from build123d import *

# Parameters (mm, degrees)
SKETCH1_W           = 12.7
SKETCH1_H           = 12.7
BOSS_EXTRUDE1_DEPTH = 2.54
FILLET1_R           = 0.635
SHELL1_START        = 0.635
SHELL1_OUTLINE_W    = 1.905
SHELL1_OUTLINE_H    = 11.43
SHELL1_DEPTH        = 11.43
SKETCH2_R           = 2.54
BOSS_EXTRUDE2_DEPTH = 1.905
BOSS_EXTRUDE3_DEPTH = 0.00254


# Read off the part's stored shape, not the designer's step: Shell1
with BuildPart() as part:
    # Sketch1 → Boss-Extrude1 (new body)
    with BuildSketch(Plane(origin=(0, 0, 0), x_dir=(1, 0, 0), z_dir=(0, 1, 0))):
        with Locations((6.35, 6.35)):
            Rectangle(SKETCH1_W, SKETCH1_H)
    extrude(amount=BOSS_EXTRUDE1_DEPTH)

    # Fillet1
    fillet1_edges = [part.edges().sort_by_distance(p)[0] for p in [
        (0, 1.27, -12.7),
        (12.7, 1.27, -12.7),
        (12.7, 1.27, 0),
        (0, 1.27, 0),
    ]]
    fillet(fillet1_edges, radius=FILLET1_R)

    # Shell1 outline → Shell1 (cut)
    with BuildSketch(Plane.YZ.offset(SHELL1_START)):
        with Locations((0.9525, -6.35)):
            Rectangle(SHELL1_OUTLINE_W, SHELL1_OUTLINE_H)
    extrude(amount=SHELL1_DEPTH, mode=Mode.SUBTRACT)

    # Sketch2 → Boss-Extrude2 (add)
    with BuildSketch(Plane(origin=(0, 1.905, 0), x_dir=(-1, 0, 0), z_dir=(0, -1, 0))):
        with Locations(Location((-6.35, 6.35, 0), (0, 0, 270))):
            Circle(SKETCH2_R)
    extrude(amount=BOSS_EXTRUDE2_DEPTH)

    # Sketch3 → Boss-Extrude3 (add)
    with BuildSketch(Plane(origin=(0, 2.54, 0), x_dir=(1, 0, 0), z_dir=(0, 1, 0))):
        Polygon((4.927762821, 8.001), (5.561872396, 8.001), (6.128564103, 6.887333133), (6.695255809, 8.001), (7.329365385, 8.001), (6.4135, 6.201070112), (6.4135, 4.826), (5.843628205, 4.826), (5.843628205, 6.201070112), align=None)
    extrude(amount=BOSS_EXTRUDE3_DEPTH)


solid = part.part
CAD build for the part. Positions are in the model's coordinates, mm. A direction names the side the tool comes from. Coordinates: 2 decimals unless noted, no trailing zeros. Write each loop counter-clockwise with the first axis right and the second up, starting at its lowest first coordinate (ties: lowest second). Pieces come first, ordered by that corner, then holes. Notation, with made-up numbers: (10, 35) - (38, 35) arc R19 cw to (38, 59) - close; hole circle Ø7 at (28.25, 32.5). An arc over 180 degrees is marked (long way). Use a Markdown table: item, result. Add a question column.
Item 1: Band-saw the part on B-B, the plane x = 2.5. Give the cut face in (y, z) (3 decimals), and give its area (3 significant figures).
Item 2: Band-saw the part on A-A, the plane z = -11. Give the cut face in (x, y) (3 decimals).
Item 3: Drill centre lines: L1, parallel to X at y = 1.6, z = -6.25 (3 decimals); L2, parallel to X at y = 1.35, z = -3 (3 decimals); L3, parallel to X at y = 1.7, z = -4.5 (3 decimals). Where is each one in solid material? Low to high. Write a range as from..to.
Item 4: Band-saw the part on D-D, the plane x = 4.75. Give the cut face in (y, z) (3 decimals), and give its area (3 significant figures).
Item 5: Mould opens along Z. For faces 1 (the face through (5.8, 0, -0.3)), 2 (the face through (5, 1.905, -9)), 3 (the face through (6, 1, 0)) say: pulls with the +Z half, pulls with the -Z half, needs draft (parallel to the pull), parting line crosses it, or undercut.
Item 6: 3-axis set-ups, long thin cutter, end or side, ignore diameter. For faces 4 (the face through (12.7, 1, -6)), 5 (the face through (8.83, 0.97, -6.9)): which of +Z, -Z, +X, -X, +Y, -Y reach the whole face in a straight line?
Item 7: Flat gauge pins, fed straight in: pin 1 (6 mm diameter, centred on x = 10.5, z = -9, fed in from +Y); pin 2 (1 mm diameter, centred on x = 10, z = -5, fed in from -Y) (3 decimals). Where does each tip first touch, or does it go through?
Item 8: Band-saw the part on C-C, the plane z = -4. Give the cut face in (x, y) (3 decimals).
Numbers:
| question | item | result |
|---|---|---|
| 1 | outline | (0, -12.7) - (2.54, -12.7) - (2.54, 0) - (0, 0) - (0, -0.635) - (1.905, -0.635) - (1.905, -12.065) - (0, -12.065) - close |
| 1 | area | 10.5 mm2 |
| 2 | outline | (0, 0) - (0.635, 0) - (0.635, 1.905) - (12.065, 1.905) - (12.065, 0) - (12.7, 0) - (12.7, 2.54) - (0, 2.54) - close |
| 3 | L1 | 0..0.635, 3.812..8.888, 12.065..12.7 |
| 3 | L2 | 0..0.635, 12.065..12.7 |
| 3 | L3 | 0..0.635, 4.61..8.09, 12.065..12.7 |
| 4 | outline | (0, -12.7) - (2.54, -12.7) - (2.54, 0) - (0, 0) - (0, -0.635) - (1.905, -0.635) - (1.905, -4.377) - (0, -4.377) - (0, -8.323) - (1.905, -8.323) - (1.905, -12.065) - (0, -12.065) - close |
| 4 | area | 18.0 mm2 |
| 5 | face 1 | needs draft |
| 5 | face 2 | undercut |
| 5 | face 3 | pulls with the +Z half |
| 6 | face 4 | +Z, -Z, +X, +Y, -Y |
| 6 | face 5 | -Y |
| 7 | pin 1 | y = 2.54 |
| 7 | pin 2 | y = 1.905 |
| 8 | outline | (0, 0) - (0.635, 0) - (0.635, 1.905) - (5.386, 1.905) - (5.386, 0) - (7.314, 0) - (7.314, 1.905) - (12.065, 1.905) - (12.065, 0) - (12.7, 0) - (12.7, 2.54) - (0, 2.54) - close |
